Answer from the drawing. Dimensions are ordinates in mm from the lowest x, y and z of the part. A direction names the side the tool comes from. Round coordinates to 2 decimals unless told otherwise and drop trailing zeros. Loops run counter-clockwise (first coordinate to the right, second up) from the corner with the lowest first, then second, coordinate; pieces in that order, holes last. Notation, with made-up numbers: M -12.75,87.25 L 1.25,87.25 A20 cw 1.25,106.25 Z; hole C 54.5,73.25 d5. An arc over 180 degrees is marked long. Answer as a JSON object with one key per item and string values.
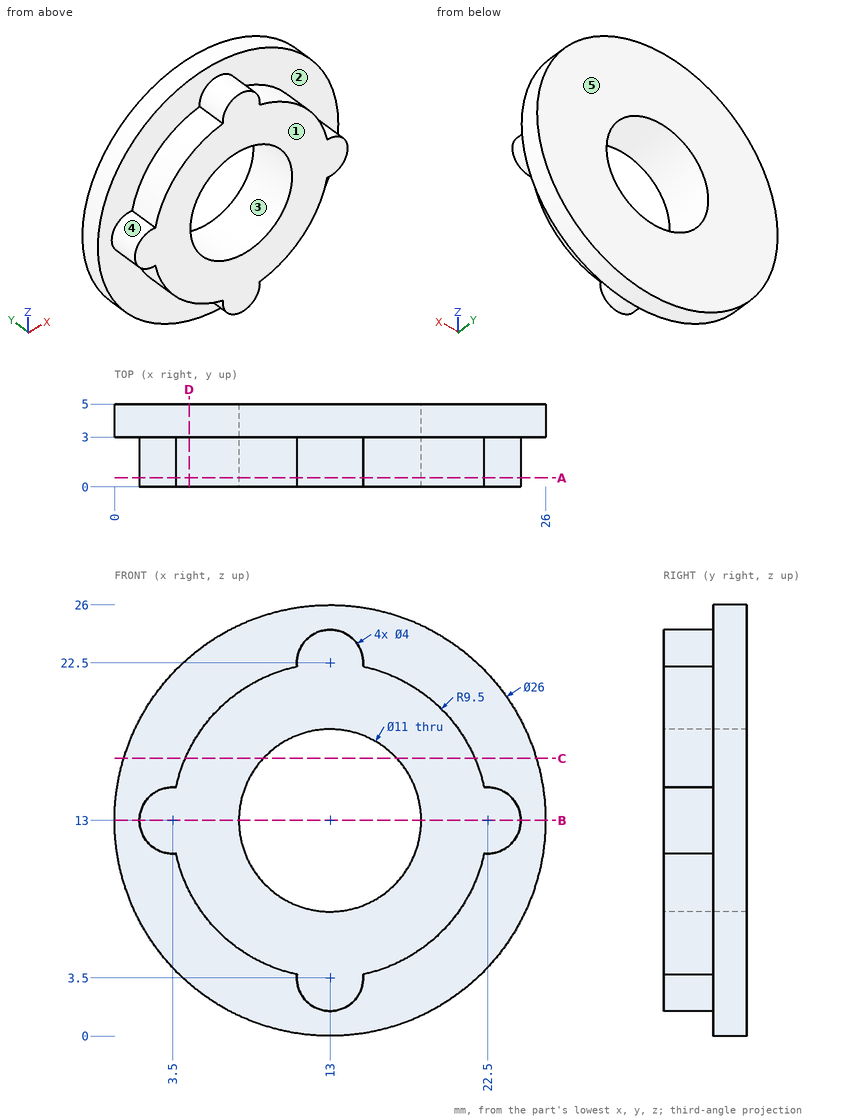
Item 1: Flat-ended cylindrical pins translate along their axes: P1, Ø1.5, axis at y = 2.5, z = 5, coming from the +X side; P2, Ø2, axis at x = 9.5, y = 4, coming from the -Z side. Find the tip coordinate at first contact, or state that the pin passes through.
Values follow:
{"P1": "x = 23.66", "P2": "z = 0.24"}
Item 2: The part is cut by section A-A (y = 0.55). Give the vertices of the cut face in (x, z), then the cut area to 3 significant figures.
Values follow:
{"outline": "M 3.71,11.01 A9.5 ccw 11.01,3.71 A2 ccw long 14.99,3.71 A9.5 ccw 22.29,11.01 A2 ccw long 22.29,14.99 A9.5 ccw 14.99,22.29 A2 ccw long 11.01,22.29 A9.5 ccw 3.71,14.99 A2 ccw long Z; hole C 13,13 d11", "area": "215 mm^2"}
Item 3: Which of the six approach directions +Z, -Z, +X, -X, +Y, -Y give full straight-line access (tool end or side, diameter ignored) to the marked faces 1 and 2?
Values follow:
{"face 1": "+Z, -Z, +X, -X, -Y", "face 2": "-Y"}
Item 4: The part is cut by section B-B (z = 13). Give the vertices of the cut face in (x, y), then the cut area to 3 significant figures.
Values follow:
{"outline": "M 0,3 L 1.5,3 L 1.5,0 L 7.5,0 L 7.5,5 L 0,5 Z; M 18.5,0 L 24.5,0 L 24.5,3 L 26,3 L 26,5 L 18.5,5 Z", "area": "66.0 mm^2"}
Item 5: Determine the mould class of the marked faces 3, 4 and 5 for opening direction Z: released by +Z, released by -Z, zero draft, split by the parting line, or undercut.
Values follow:
{"face 3": "undercut", "face 4": "split by the parting line", "face 5": "zero draft"}
Item 6: The part is cut by section D-D (x = 4.5). Give the vertices of the cut face in (y, z).
Values follow:
{"outline": "M 0,8.76 L 3,8.76 L 3,3.16 L 5,3.16 L 5,22.84 L 3,22.84 L 3,17.24 L 0,17.24 Z"}
Item 7: The part is cut by section C-C (z = 16.75). Give the vertices of the cut face in (x, y), then the cut area to 3 significant figures.
Values follow:
{"outline": "M 0.55,3 L 4.27,3 L 4.27,0 L 8.98,0 L 8.98,5 L 0.55,5 Z; M 17.02,0 L 21.73,0 L 21.73,3 L 25.45,3 L 25.45,5 L 17.02,5 Z", "area": "61.9 mm^2"}
Item 8: Straight lines are drawn through the part: line 1 (Z direction, x = 13, y = 2.6); line 2 (X direction, y = 4.65, z = 12.75); line 3 (Y direction, x = 21.75, z = 6). For each, find the intervals that lie inside material, in ascending order.
Values follow:
{"line 1": "1.5 to 7.5, 18.5 to 24.5", "line 2": "0 to 7.51, 18.49 to 26", "line 3": "3 to 5"}
